Part model, mm, in its own coordinate system. Coordinates: 2 decimals unless noted, no trailing zeros. Order: outer loops, then holes, each group sorted by start corner. A loop starts at its lowest first (then second) coordinate and runs counter-clockwise, first axis right, second up.
Autodesk Inventor part; units mm, degrees
ref_plane "YZ Plane" through (0, 0, 0) normal (1, 0, 0) x (0, 1, 0)
ref_plane "XZ Plane" through (0, 0, 0) normal (0, 1, 0) x (-1, 0, 0)
ref_plane "XY Plane" through (0, 0, 0) normal (0, 0, 1) x (1, 0, 0)
sketch "main" plane through (0, 0, 0) normal (0, 0, 1) x (1, 0, 0)
  circle A0 centre (31.5379, -87.1249) radius 2.0955
  circle A1 centre (8.5185, -76.3887) radius 2.0955
  line L0 (52.8956, -28.6403) -> (-10.6273, 2.6327)
  circle A2 centre (1.6034, -31.1233) radius 2.1844
  arc A3 (-63.4783, 65.8273) -> (-10.6273, 2.6327) centre (34.3111, 93.9132) ccw
  line L1 (-57.9066, -8.669) -> (-22.6804, -8.669)
  circle A4 centre (59.152, -57.9639) radius 2.1844
  line L2 (59.4746, -36.466) -> (65.2461, -56.1797)
  arc A5 (63.7627, -62.3301) -> (65.2461, -56.1797) centre (59.152, -57.9639) ccw
  line L3 (-64.2566, 65.7178) -> (-64.2566, -2.319)
  line L4 (-64.2566, 68.6882) -> (6.9552, 68.6882) construction
  arc A6 (-64.2566, -2.319) -> (-57.9066, -8.669) centre (-57.9066, -2.319) ccw
  circle A7 centre (20.0282, -81.7568) radius 2.0955
  arc A8 (28.8539, -92.8798) -> (36.1487, -91.4911) centre (31.5379, -87.1249) ccw
  line L5 (28.8539, -92.8798) -> (5.8344, -82.1435)
  line L6 (36.1487, -91.4911) -> (63.7627, -62.3301)
  circle A9 centre (47.6422, -52.5958) radius 2.2479
  arc A10 (-63.4783, 65.8273) -> (-64.2566, 65.7178) centre (-63.8597, 65.7178) ccw
  arc A11 (59.4746, -36.466) -> (52.8956, -28.6403) centre (47.2862, -40.0344) ccw
  circle A12 centre (36.1325, -47.2277) radius 2.1844
  arc A13 (-3.8107, -27.7809) -> (-4.6861, -32.0859) centre (1.6034, -31.1233) ccw
  line L7 (-3.8107, -27.7809) -> (-3.8107, -27.7809)
  line L8 (-5.8782, -19.0419) -> (-22.6804, -8.669)
  arc A14 (-3.8107, -27.7809) -> (-5.8782, -19.0419) centre (-9.2139, -24.4452) ccw
  circle A15 centre (-61.0816, 50.233) radius 2.0955
  circle A16 centre (-57.9066, -2.319) radius 2.0955
  arc A17 (2.2416, -77.3494) -> (5.8344, -82.1435) centre (8.5185, -76.3887) ccw
  line L9 (2.2416, -77.3494) -> (-4.6861, -32.0859)
  point P0 (22.7298, -27.8341)
  point P1 (-67.4316, 93.9132)
  point P2 (-64.2566, -8.669)
  point P3 (57.9062, -31.1089)
  point P4 (57.9062, -31.1089)
  point P5 (-0.4749, -22.3776)
  point P6 (-1.0693, -36.8975)
  dimension "d4" = 12.7
  dimension "d5" = 4.191
  dimension "d6" = 25.4
  dimension "d10" = 6.35
  dimension "d11" = 4.191
  dimension "d12" = 12.7
  dimension "d14" = 4.4958
  dimension "d23" = 0.3969
  dimension "d25" = 12.7
  dimension "d26" = 12.7
  dimension "d27" = 4.3688
  dimension "d28" = 6.35
  dimension "d29" = 6.35
  dimension "d31" = 4.191
  dimension "d33" = 4.191
  dimension "d35" = 12.7
  dimension "d36" = 12.7
  dimension "d37" = 38.1
  dimension "d38" = 12.7
sketch "Sketch1" plane through (0, 0, 0) normal (1, 0, 0) x (0, 1, 0)
  circle A0 centre (31.5379, -87.1249) radius 2.0955
  circle A1 centre (8.5185, -76.3887) radius 2.0955
  line L0 (52.8956, -28.6403) -> (-10.6273, 2.6327)
  circle A2 centre (1.6034, -31.1233) radius 2.1844
  arc A3 (-63.4783, 65.8273) -> (-10.6273, 2.6327) centre (34.3111, 93.9132) ccw
  line L1 (-57.9066, -8.669) -> (-22.6804, -8.669)
  circle A4 centre (59.152, -57.9639) radius 2.1844
  line L2 (59.4746, -36.466) -> (65.2461, -56.1797)
  arc A5 (63.7627, -62.3301) -> (65.2461, -56.1797) centre (59.152, -57.9639) ccw
  line L3 (-64.2566, 65.7178) -> (-64.2566, -2.319)
  line L4 (-64.2566, 68.6882) -> (6.9552, 68.6882) construction
  arc A6 (-64.2566, -2.319) -> (-57.9066, -8.669) centre (-57.9066, -2.319) ccw
  circle A7 centre (20.0282, -81.7568) radius 2.0955
  arc A8 (28.8539, -92.8798) -> (36.1487, -91.4911) centre (31.5379, -87.1249) ccw
  line L5 (28.8539, -92.8798) -> (5.8344, -82.1435)
  line L6 (36.1487, -91.4911) -> (63.7627, -62.3301)
  circle A9 centre (47.6422, -52.5958) radius 2.2479
  arc A10 (-63.4783, 65.8273) -> (-64.2566, 65.7178) centre (-63.8597, 65.7178) ccw
  arc A11 (59.4746, -36.466) -> (52.8956, -28.6403) centre (47.2862, -40.0344) ccw
  circle A12 centre (36.1325, -47.2277) radius 2.1844
  arc A13 (-3.8107, -27.7809) -> (-4.6861, -32.0859) centre (1.6034, -31.1233) ccw
  line L7 (-3.8107, -27.7809) -> (-3.8107, -27.7809)
  line L8 (-5.8782, -19.0419) -> (-22.6804, -8.669)
  arc A14 (-3.8107, -27.7809) -> (-5.8782, -19.0419) centre (-9.2139, -24.4452) ccw
  circle A15 centre (-61.0816, 50.233) radius 2.0955
  circle A16 centre (-57.9066, -2.319) radius 2.0955
  arc A17 (2.2416, -77.3494) -> (5.8344, -82.1435) centre (8.5185, -76.3887) ccw
  line L9 (2.2416, -77.3494) -> (-4.6861, -32.0859)
  point P0 (0, 0)
extrude "Extrusion2" add sketch "Sketch1" along normal blind 1.5875
sketch "Sketch2" plane through (1.5875, 0, 0) normal (1, 0, 0) x (0, 0, -1)
  line L0 (82.1435, 5.8344) -> (92.8798, 28.8539)
  arc A0 (77.3494, 2.2416) -> (82.1435, 5.8344) centre (76.3887, 8.5185) ccw
  line L1 (91.4911, 36.1487) -> (62.3301, 63.7627)
  arc A1 (92.8798, 28.8539) -> (91.4911, 36.1487) centre (87.1249, 31.5379) ccw
  circle A2 centre (57.9639, 59.152) radius 2.1844
  arc A3 (63.7193, 56.469) -> (62.3301, 63.7627) centre (57.9639, 59.152) ccw
  circle A4 centre (31.1233, 1.6034) radius 2.1844
  arc A5 (32.0859, -4.6861) -> (36.8902, -1.0849) centre (31.1233, 1.6034) ccw
  line L2 (63.7193, 56.469) -> (36.8902, -1.0849)
  line L3 (32.0859, -4.6861) -> (77.3494, 2.2416)
  point P0 (0, 0)
extrude "Extrusion3" cut sketch "Sketch2" against normal blind 25.4 contours A0 L3 A5 L2 A3 L1 A1 L0
equation "\"BendRadius\" = Thickness"
equation "\"BendReliefWidth\" = Thickness"
equation "\"BendReliefDepth\" = 0.5 * Thickness"
equation "\"CornerReliefSize\" = 4 * Thickness"
equation "\"MinimumRemnant\" = 2 * Thickness"
equation "\"TransitionRadius\" = BendRadius"
equation "\"JacobiRadiusSize\" = BendRadius"
equation "\"GapSize\" = Thickness"
properties part number "Ramp" material "Acetal Resin, White"
(1) Slice it at D-D, the plane z = 55.5. Give the cut face in (x, y).
(2) Probe line 1 (Z direction, x = 0.1, y = 36.5); line 2 (Z direction, x = 1.5, y = 38); line 3 (Y direction, x = 0.8, z = 35.5). List the from-to ranges inside material, lowest first.
(3) Slice it at B-B, the plane y = 36. Give the cut face in (x, z).
(4) Pull direction Y, two halves, no side cores. Call faces 1 (the face through (0.78, 1.13, -28.99)), 2 (the face through (0.78, 62.32, -46.18)), 3 (the face through (1.588, -4, -13)): +Y half, -Y half, draft (parallel to the pull), parting line (faces both ways), or undercut.
(5) Slice it at C-C, the plane y = 10. Give the cut face in (x, z).
(6) Slice it at A-A, the plane x = 1.15. Give the cut face in (y, z), then the cut area to 3 significant figures.
Here are the results:
1. outline: (0, -64.26) - (1.59, -64.26) - (1.59, -59.9) - (0, -59.9) - close
2. line 1: z = -54.41 to -49.38, -45.07 to -20.57
2. line 2: z = -55.11 to -48.36, -46.09 to -21.31
2. line 3: y = -64.26 to -48.99
3. outline: (0, -54.18) - (1.59, -54.18) - (1.59, -49.41) - (0, -49.41) - close; (0, -45.05) - (1.59, -45.05) - (1.59, -20.32) - (0, -20.32) - close
4. face 1: undercut
4. face 2: +Y half
4. face 3: draft
5. outline: (0, -42.06) - (1.59, -42.06) - (1.59, -7.52) - (0, -7.52) - close
6. outline: (-64.26, -2.32) arc R6.35 ccw to (-57.91, -8.67) - (-22.68, -8.67) - (-5.88, -19.04) arc R6.35 cw to (-3.81, -27.78) arc R6.36 ccw to (-4.69, -32.09) arc R6.36 ccw to (-1.08, -36.89) - (56.47, -63.72) arc R6.35 ccw to (63.76, -62.33) arc R6.35 ccw to (65.25, -56.18) - (59.47, -36.47) arc R12.7 ccw to (52.9, -28.64) - (-10.63, 2.63) arc R101.74 cw to (-63.48, 65.83) arc R0.4 ccw to (-64.26, 65.72) - close; hole circle Ø4.19 at (-61.08, 50.23); hole circle Ø4.19 at (-57.91, -2.32); hole circle Ø4.37 at (1.6, -31.12); hole circle Ø4.37 at (36.13, -47.23); hole circle Ø4.5 at (47.64, -52.6); hole circle Ø4.37 at (59.15, -57.96)
6. area: 4,170 mm2
